from build123d import *

# Parameters (mm, degrees)
SKETCH1_R               = 22.5
SKETCH1_R_2             = 20.5
EXTRUDE1_DEPTH          = 500
SKETCH2_R               = 22.5
EXTRUDE2_DEPTH          = 20
SKETCH3_R               = 22.5
EXTRUDE3_DEPTH          = 20
SKETCH5_W               = 3
SKETCH5_H               = 36.728735344
EXTRUDE4_DEPTH          = 30
SKETCH7_W               = 3
SKETCH7_H               = 36.728735344
EXTRUDE6_DEPTH          = 30
SKETCH8_R               = 5
CUT_EXTRUDE1_DEPTH      = 10.5
CUT_EXTRUDE1_DEPTH_BACK = 36.5
SKETCH9_R               = 5
CUT_EXTRUDE2_DEPTH      = 10.5
CUT_EXTRUDE2_DEPTH_BACK = 36.5


with BuildPart() as part:
    # Sketch1 → Extrude1 (new body)
    with BuildSketch(Plane(origin=(0, 0, 0), x_dir=(1, 0, 0), z_dir=(0, 1, 0))):
        with Locations(Location((0, 0, 0), (0, 0, 270))):  # turned: the seam where the file's is
            Circle(SKETCH1_R)
        with Locations(Location((0, 0, 0), (0, 0, 270))):  # turned: the seam where the file's is
            Circle(SKETCH1_R_2, mode=Mode.SUBTRACT)
    extrude(amount=EXTRUDE1_DEPTH)

    # Sketch2 → Extrude2 (add)
    with BuildSketch(Plane(origin=(0, 500, 0), x_dir=(-1, 0, 0), z_dir=(0, 1, 0))):
        with Locations(Location((0, 0, 0), (0, 0, 90))):  # turned: the seam where the file's is
            Circle(SKETCH2_R)
    extrude(amount=EXTRUDE2_DEPTH)

    # Sketch3 → Extrude3 (add)
    with BuildSketch(Plane.XZ):
        with Locations(Location((0, 0, 0), (0, 0, 270))):  # turned: the seam where the file's is
            Circle(SKETCH3_R)
    extrude(amount=EXTRUDE3_DEPTH)

    # Sketch5 → Extrude4 (add)
    with BuildSketch(Plane.XZ.offset(20)):
        with Locations((-11.5, 0)):
            Rectangle(SKETCH5_W, SKETCH5_H)
        with Locations((11.5, 0)):
            Rectangle(SKETCH5_W, SKETCH5_H)
    extrude(amount=EXTRUDE4_DEPTH)

    # Sketch7 → Extrude6 (add)
    with BuildSketch(Plane(origin=(0, 520, 0), x_dir=(-1, 0, 0), z_dir=(0, 1, 0))):
        with Locations((-11.5, 0)):
            Rectangle(SKETCH7_W, SKETCH7_H)
        with Locations((11.5, 0)):
            Rectangle(SKETCH7_W, SKETCH7_H)
    extrude(amount=EXTRUDE6_DEPTH)

    # Sketch8 → Cut-Extrude1 (cut, two sides)
    with BuildSketch(Plane.ZY.offset(13)) as cut_extrude1_sk:
        with Locations((0, 540)):
            Circle(SKETCH8_R)
    extrude(amount=CUT_EXTRUDE1_DEPTH, mode=Mode.SUBTRACT)
    extrude(cut_extrude1_sk.sketch, amount=-CUT_EXTRUDE1_DEPTH_BACK, mode=Mode.SUBTRACT)

    # Sketch9 → Cut-Extrude2 (cut, two sides)
    with BuildSketch(Plane.ZY.offset(13)) as cut_extrude2_sk:
        with Locations((0, -40)):
            Circle(SKETCH9_R)
    extrude(amount=CUT_EXTRUDE2_DEPTH, mode=Mode.SUBTRACT)
    extrude(cut_extrude2_sk.sketch, amount=-CUT_EXTRUDE2_DEPTH_BACK, mode=Mode.SUBTRACT)


solid = part.part
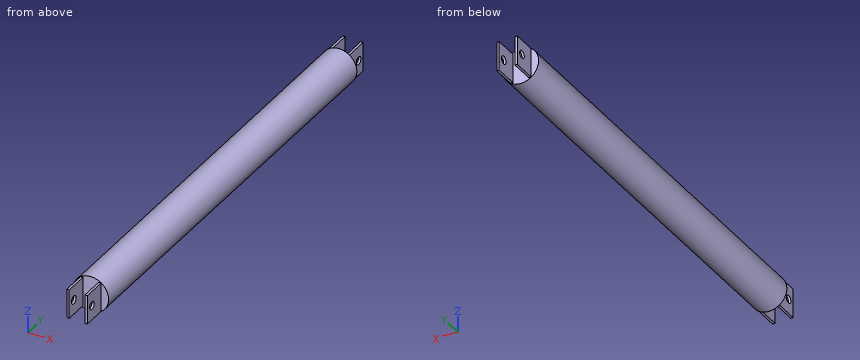
Part model, mm, in its own coordinate system. Round coordinates to 2 decimals unless told otherwise and drop trailing zeros. Write each loop counter-clockwise with the first axis right and the second up, starting at its lowest first coordinate (ties: lowest second). Pieces come first, ordered by that corner, then holes. Notation, with made-up numbers: M 4,19 L 12,19 A35 cw 12,53 Z; hole C 45.25,71 d4. An arc over 180 degrees is marked long. Return JSON: item names as keys, results as strings. Group by question number.
(1) Pin check, flat tips, straight feed: pin 1 Ø2 at (x, y) = (-8.5, 240.5) entering from +Z; pin 2 Ø12 at (x, y) = (8, 73) entering from +Z; pin 3 Ø2 at (y, z) = (30.5, 8) entering from -X. Stop position of each tip, or through.
(2) Saw through at D-D on y = 350. Write the cut outline in (x, z).
(3) Drill centre lines: probe 1 along Y at (x, z) = (11, 0); probe 2 along Y at (x, z) = (-7, 12); probe 3 along Z at (x, y) = (2, 350.5). Where is each one in solid material? Low to high.
(4) Saw through at B-B on x = 0. Write the cut outline in (y, z).
(5) Saw through at C-C on z = 0. Count the separate pieces of the cut face and the enclosed holes in it, then the cut area to 3 significant figures.
(6) Saw through at A-A on y = 540. Write the cut outline in (x, z), then the cut area to 3 significant figures.
Returned:
{
 "1": {"pin 1": "z = 21.21", "pin 2": "z = 22.41", "pin 3": "x = -21.38"},
 "2": {"outline": "C 0,0 d45; hole C 0,0 d41"},
 "3": {"probe 1": "-50 to -45, -35 to 0, 500 to 535, 545 to 550", "probe 2": "-20 to 0, 500 to 520", "probe 3": "-22.41 to -20.4, 20.4 to 22.41"},
 "4": {"outline": "M -20,-22.5 L 520,-22.5 L 520,22.5 L -20,22.5 Z; hole M 0,-20.5 L 500,-20.5 L 500,20.5 L 0,20.5 Z"},
 "5": {"separate pieces": "5", "enclosed holes": "1", "area": "4,040 mm²"},
 "6": {"outline": "M -13,-18.36 L -10,-18.36 L -10,-5 L -13,-5 Z; M -13,5 L -10,5 L -10,18.36 L -13,18.36 Z; M 10,-18.36 L 13,-18.36 L 13,-5 L 10,-5 Z; M 10,5 L 13,5 L 13,18.36 L 10,18.36 Z", "area": "160 mm²"}
}
